Could you check a few things on this model? Use its own coordinates, in mm. Coordinates: 2 decimals unless noted, no trailing zeros. Write each loop counter-clockwise with the first axis right and the second up, starting at its lowest first coordinate (ties: lowest second). Pieces come first, ordered by that corner, then holes.
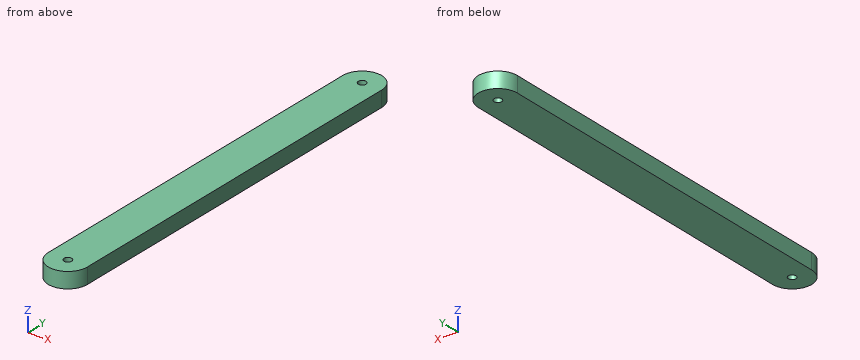
```python
from build123d import *

# Parameters (mm, degrees)
BOSS_EXTRUDE1_DEPTH              = 20
F_10_0MM_DOWEL_HOLE1_D           = 10
F_10_0MM_DOWEL_HOLE1_CSINK_D     = 10.05
F_10_0MM_DOWEL_HOLE1_CSINK_ANGLE = 90
SCALE1_SCALE                     = 0.125


with BuildPart() as part:
    # Sketch2 → Boss-Extrude1 (new body)
    with BuildSketch(Plane.XY):
        with BuildLine():
            Line((-50, -240), (-50, 240))
            ThreePointArc((-50, 240), (-25, 265), (0, 240))
            Line((0, 240), (0, -240))
            ThreePointArc((0, -240), (-25, -265), (-50, -240))
        make_face()
    extrude(amount=BOSS_EXTRUDE1_DEPTH)

    # Ø10.0mm Dowel Hole1 (through all)
    with Locations(Plane.XY.offset(20)):
        with Locations((-25, 240), (-25, -240)):
            CounterSinkHole(F_10_0MM_DOWEL_HOLE1_D / 2, F_10_0MM_DOWEL_HOLE1_CSINK_D / 2, counter_sink_angle=F_10_0MM_DOWEL_HOLE1_CSINK_ANGLE)


with BuildPart() as part_1:
    # Scale1: scaled about (-25, 0, 9.999999619)
    add(part.part.scale(SCALE1_SCALE).moved(Location((-21.875, 0, 8.749999667))))


solid = part_1.part
```
1. For pin 1 (1 mm diameter, centred on x = -25, y = 30, fed in from -Z), with a flat end and sliding along its axis, tell me the tip position at first contact or that it passes through.
Verdict:
pin 1: passes through
2. I want a section at B-B on z = 10.15. Please give me the cut outline in (x, y) (3 decimals).
Verdict:
outline: (-28.125, -30) arc R3.125 ccw to (-21.875, -30) - (-21.875, 30) arc R3.125 ccw to (-28.125, 30) - close; hole circle Ø1.25 at (-25, -30); hole circle Ø1.25 at (-25, 30)
3. I want a section at A-A on x = -25. Please give me the cut outline in (y, z) (3 decimals), plus the area to 3 significant figures.
Verdict:
outline: (-33.125, 8.75) - (-30.625, 8.75) - (-30.625, 11.247) - (-30.628, 11.25) - (-33.125, 11.25) - close; (-29.375, 8.75) - (29.375, 8.75) - (29.375, 11.247) - (29.372, 11.25) - (-29.372, 11.25) - (-29.375, 11.247) - close; (30.625, 8.75) - (33.125, 8.75) - (33.125, 11.25) - (30.628, 11.25) - (30.625, 11.247) - close
area: 159 mm2
4. Please list where these lines run through material, in increasing order: line 1 along Y through (x, z) = (-25, 10.1) (3 decimals); line 2 along X through (y, z) = (30, 10.5) (3 decimals); line 3 along Y through (x, z) = (-24.5, 10.35) (3 decimals).
Verdict:
line 1: y = -33.125 to -30.625, -29.375 to 29.375, 30.625 to 33.125
line 2: x = -28.125 to -25.625, -24.375 to -21.875
line 3: y = -33.085 to -30.375, -29.625 to 29.625, 30.375 to 33.085
